For this review, take the finished solid that the model builds, in its own axes (mm). A direction names the side the tool comes from. Coordinates: 2 decimals unless noted, no trailing zeros. Write each loop counter-clockwise with the first axis right and the second up, starting at its lowest first coordinate (ties: lowest second). Pieces come first, ordered by that corner, then holes. Notation, with made-up numbers: M 37,-30.5 L 44,-30.5 A6 cw 44,-21.5 Z; hole C 79.25,55.5 d6. An arc over 180 degrees is marked long. One line per question, with ' | ' between items.
from build123d import *

# Parameters (mm, degrees)
SKETCH1_W           = 200
SKETCH1_H           = 194
BOSS_EXTRUDE1_DEPTH = 8
SKETCH4_R           = 2.4
CUT_EXTRUDE1_DEPTH  = 6
SKETCH5_W           = 200
SKETCH5_H           = 194
SKETCH5_W_2         = 192
SKETCH5_H_2         = 180
BOSS_EXTRUDE4_DEPTH = 60
SKETCH6_W           = 192
SKETCH6_H           = 6
BOSS_EXTRUDE5_DEPTH = 4
SKETCH7_R           = 2.4
CUT_EXTRUDE2_DEPTH  = 6
SKETCH10_R          = 3.9
SKETCH10_R_2        = 7.7
SKETCH10_W          = 12.3
SKETCH10_H          = 19
CUT_EXTRUDE4_DEPTH  = 10
SKETCH16_R          = 5
SKETCH16_R_2        = 5.9
SKETCH16_W          = 13
SKETCH16_H          = 16
CUT_EXTRUDE5_DEPTH  = 10
SKETCH17_W          = 15
SKETCH17_H          = 15
CUT_EXTRUDE6_DEPTH  = 3
SKETCH19_R          = 2.4
CUT_EXTRUDE7_DEPTH  = 5
SKETCH20_R          = 6.5
CUT_EXTRUDE8_DEPTH  = 6
SKETCH22_W          = 35
SKETCH22_H          = 34
CUT_EXTRUDE9_DEPTH  = 4
SKETCH23_W          = 34.5
SKETCH23_H          = 19.9
CUT_EXTRUDE10_DEPTH = 12
CUT_EXTRUDE11_DEPTH = 1
SKETCH25_R          = 2.4
CUT_EXTRUDE12_DEPTH = 5
SKETCH26_W          = 144
SKETCH26_H          = 60
CUT_EXTRUDE13_DEPTH = 287.810041665
SKETCH27_W          = 42.5
SKETCH27_H          = 27.9
SKETCH27_W_2        = 34.5
SKETCH27_H_2        = 19.9
BOSS_EXTRUDE7_DEPTH = 1
FILLET5_R           = 5
BOSS_EXTRUDE8_DEPTH = 3
FILLET6_R           = 5
SKETCH30_R          = 2.4
CUT_EXTRUDE14_DEPTH = 5
SKETCH32_R          = 1.65
CUT_EXTRUDE15_DEPTH = 15
FILLET7_R           = 5
FILLET8_R           = 5
FILLET9_R           = 5
FILLET10_R          = 25
SKETCH33_W          = 206
SKETCH33_H          = 200
BOSS_EXTRUDE9_DEPTH = 5


with BuildPart() as part:
    # Sketch1 → Boss-Extrude1 (new body)
    with BuildSketch(Plane(origin=(0, 0, 0), x_dir=(1, 0, 0), z_dir=(0, 1, 0))):
        with Locations((100, -97)):
            Rectangle(SKETCH1_W, SKETCH1_H)
    extrude(amount=BOSS_EXTRUDE1_DEPTH)

    # Sketch4 → Cut-Extrude1 (cut)
    with BuildSketch(Plane(origin=(0, 8, 0), x_dir=(1, 0, 0), z_dir=(0, 1, 0))):
        with Locations(Location((9.25, -31.25, 0), (0, 0, 270))):
            Circle(SKETCH4_R)
        with Locations(Location((95.25, -31.25, 0), (0, 0, 270))):
            Circle(SKETCH4_R)
        with Locations(Location((95.25, -162.75, 0), (0, 0, 90))):
            Circle(SKETCH4_R)
        with Locations(Location((9.25, -162.75, 0), (0, 0, 90))):
            Circle(SKETCH4_R)
        with Locations(Location((190.75, -162.75, 0), (0, 0, 270))):
            Circle(SKETCH4_R)
        with Locations(Location((104.75, -162.75, 0), (0, 0, 270))):
            Circle(SKETCH4_R)
        with Locations(Location((104.75, -31.25, 0), (0, 0, 90))):
            Circle(SKETCH4_R)
        with Locations(Location((190.75, -31.25, 0), (0, 0, 90))):
            Circle(SKETCH4_R)
    extrude(amount=-CUT_EXTRUDE1_DEPTH, mode=Mode.SUBTRACT)

    # Sketch5 → Boss-Extrude4 (add)
    with BuildSketch(Plane(origin=(0, 8, 0), x_dir=(1, 0, 0), z_dir=(0, 1, 0))):
        with Locations((100, -97)):
            Rectangle(SKETCH5_W, SKETCH5_H)
        with Locations((100, -97)):
            Rectangle(SKETCH5_W_2, SKETCH5_H_2, mode=Mode.SUBTRACT)
    extrude(amount=BOSS_EXTRUDE4_DEPTH)

    # Sketch6 → Boss-Extrude5 (add)
    with BuildSketch(Plane.XY.offset(7)):
        with Locations((100, 65)):
            Rectangle(SKETCH6_W, SKETCH6_H)
    boss_extrude5 = extrude(amount=BOSS_EXTRUDE5_DEPTH)

    # Sketch7 → Cut-Extrude2 (cut)
    with BuildSketch(Plane(origin=(0, 68, 0), x_dir=(1, 0, 0), z_dir=(0, 1, 0))):
        with Locations(Location((12.5, -4, 0), (0, 0, 270))):
            Circle(SKETCH7_R)
        with Locations(Location((62.5, -4, 0), (0, 0, 270))):
            Circle(SKETCH7_R)
        with Locations(Location((187.5, -4, 0), (0, 0, 270))):
            Circle(SKETCH7_R)
        with Locations(Location((137.5, -4, 0), (0, 0, 270))):
            Circle(SKETCH7_R)
    cut_extrude2 = extrude(amount=-CUT_EXTRUDE2_DEPTH, mode=Mode.SUBTRACT)

    # Mirror3: Boss-Extrude5 across plane
    add(boss_extrude5.mirror(Plane.XY.offset(97)))

    # Mirror5: Cut-Extrude2 across plane
    add(cut_extrude2.mirror(Plane.XY.offset(97)), mode=Mode.SUBTRACT)

    # Sketch10 → Cut-Extrude4 (cut)
    with BuildSketch(Plane.XY.offset(194)):
        with Locations((18.85, 20)):
            Circle(SKETCH10_R)
        with Locations((170, 32)):
            Circle(SKETCH10_R_2)
        with Locations((40, 20)):
            Rectangle(SKETCH10_W, SKETCH10_H)
    extrude(amount=-CUT_EXTRUDE4_DEPTH, mode=Mode.SUBTRACT)

    # Sketch16 → Cut-Extrude5 (cut)
    with BuildSketch(Plane(origin=(0, 0, 0), x_dir=(-1, 0, 0), z_dir=(0, 0, -1))):
        with Locations((-53, 48)):
            Circle(SKETCH16_R)
        with Locations((-63.5, 37.5)):
            Circle(SKETCH16_R)
        with Locations((-42.5, 37.5)):
            Circle(SKETCH16_R)
        with Locations((-53, 27)):
            Circle(SKETCH16_R)
        with Locations((-18, 48)):
            Circle(SKETCH16_R_2)
        with Locations((-82.2, 42.6)):
            Rectangle(SKETCH16_W, SKETCH16_H)
    extrude(amount=-CUT_EXTRUDE5_DEPTH, mode=Mode.SUBTRACT)

    # Sketch17 → Cut-Extrude6 (cut)
    with BuildSketch(Plane(origin=(0, 0, 0), x_dir=(-1, 0, 0), z_dir=(0, 0, -1))):
        with Locations((-18, 48)):
            Rectangle(SKETCH17_W, SKETCH17_H)
    extrude(amount=-CUT_EXTRUDE6_DEPTH, mode=Mode.SUBTRACT)

    # Sketch19 → Cut-Extrude7 (cut)
    with BuildSketch(Plane.XY.offset(7)):
        with Locations((32.5, 54.4)):
            Circle(SKETCH19_R)
        with Locations((92.5, 54.4)):
            Circle(SKETCH19_R)
        with Locations((92.5, 17.6)):
            Circle(SKETCH19_R)
        with Locations((32.5, 17.6)):
            Circle(SKETCH19_R)
    extrude(amount=-CUT_EXTRUDE7_DEPTH, mode=Mode.SUBTRACT)

    # Sketch20 → Cut-Extrude8 (cut)
    with BuildSketch(Plane.XY.offset(7)):
        with Locations((53, 48)):
            Circle(SKETCH20_R)
        with Locations((42.5, 37.5)):
            Circle(SKETCH20_R)
        with Locations((53, 27)):
            Circle(SKETCH20_R)
        with Locations((63.5, 37.5)):
            Circle(SKETCH20_R)
    extrude(amount=-CUT_EXTRUDE8_DEPTH, mode=Mode.SUBTRACT)

    # Sketch22 → Cut-Extrude9 (cut)
    with BuildSketch(Plane.XY.offset(7)):
        with Locations((163.5, 35.101020514)):
            Rectangle(SKETCH22_W, SKETCH22_H)
    extrude(amount=-CUT_EXTRUDE9_DEPTH, mode=Mode.SUBTRACT)

    # Sketch23 → Cut-Extrude10 (cut)
    with BuildSketch(Plane.XY.offset(3)):
        with Locations((163.5, 36.051020514)):
            Rectangle(SKETCH23_W, SKETCH23_H)
    extrude(amount=-CUT_EXTRUDE10_DEPTH, mode=Mode.SUBTRACT)

    # Sketch24 → Cut-Extrude11 (cut)
    with BuildSketch(Plane.XY.offset(3)):
        Polygon((146.25, 26.101020514), (146.25, 22.001020514), (153.5, 22.001020514), (153.5, 18.101020514), (173.5, 18.101020514), (173.5, 22.001020514), (180.75, 22.001020514), (180.75, 26.101020514), align=None)
    extrude(amount=-CUT_EXTRUDE11_DEPTH, mode=Mode.SUBTRACT)

    # Sketch25 → Cut-Extrude12 (cut)
    with BuildSketch(Plane.XY.offset(7)):
        with Locations((141, 37.101020514)):
            Circle(SKETCH25_R)
        with Locations((186, 37.101020514)):
            Circle(SKETCH25_R)
    extrude(amount=-CUT_EXTRUDE12_DEPTH, mode=Mode.SUBTRACT)

    # Sketch26 → Cut-Extrude13 (cut, through all)
    with BuildSketch(Plane.ZY):
        with Locations((97, 38)):
            Rectangle(SKETCH26_W, SKETCH26_H)
    extrude(amount=-CUT_EXTRUDE13_DEPTH, mode=Mode.SUBTRACT)

    # Sketch27 → Boss-Extrude7 (add)
    with BuildSketch(Plane(origin=(0, 0, 0), x_dir=(-1, 0, 0), z_dir=(0, 0, -1))):
        with Locations((-163.5, 36.051020514)):
            Rectangle(SKETCH27_W, SKETCH27_H)
        with Locations((-163.5, 36.051020514)):
            Rectangle(SKETCH27_W_2, SKETCH27_H_2, mode=Mode.SUBTRACT)
    extrude(amount=BOSS_EXTRUDE7_DEPTH)

    # Fillet5
    fillet5_edges = [part.edges().sort_by_distance(p)[0] for p in [
        (184.75, 50.001020514, -0.5),
        (184.75, 22.101020514, -0.5),
        (142.25, 22.101020514, -0.5),
        (142.25, 50.001020514, -0.5),
    ]]
    fillet(fillet5_edges, radius=FILLET5_R)

    # Sketch28 → Boss-Extrude8 (add)
    with BuildSketch(Plane.ZY.offset(-196)):
        Polygon((25, 68), (11, 68), (11, 62), (7, 62), (7, 38), (11, 38), (25, 38), align=None)
        Polygon((183, 68), (169, 68), (169, 38), (183, 38), (187, 38), (187, 62), (183, 62), align=None)
    boss_extrude8 = extrude(amount=BOSS_EXTRUDE8_DEPTH)

    # Fillet6
    # the kernel refuses this fillet: 5 mm, written as the material it adds along each edge
    with BuildSketch(Plane(origin=(196, 38, 169), x_dir=(-1, 0, 0), z_dir=(0, 0, 1)), Plane(origin=(196, 38, 7), x_dir=(-1, 0, 0), z_dir=(0, 0, 1))) as fillet6_piece_1:
        with BuildLine():
            CenterArc((5, 4.582575695), FILLET6_R, 180, 66.421821522)
            Line((0, 4.582575695), (0, 0))
            Line((0, 0), (3, 0))
        make_face()
    extrude(amount=18)

    # Sketch30 → Cut-Extrude14 (cut)
    with BuildSketch(Plane.ZY.offset(-193)):
        with Locations((18, 60)):
            Circle(SKETCH30_R)
        with Locations((18, 44)):
            Circle(SKETCH30_R)
        with Locations(Location((176, 44, 0), (0, 0, 180))):
            Circle(SKETCH30_R)
        with Locations(Location((176, 60, 0), (0, 0, 180))):
            Circle(SKETCH30_R)
    cut_extrude14 = extrude(amount=-CUT_EXTRUDE14_DEPTH, mode=Mode.SUBTRACT)

    # Sketch32 → Cut-Extrude15 (cut)
    with BuildSketch(Plane.ZY.offset(-198)):
        with Locations((18, 60)):
            Circle(SKETCH32_R)
        with Locations((18, 44)):
            Circle(SKETCH32_R)
        with Locations((176, 44)):
            Circle(SKETCH32_R)
        with Locations((176, 60)):
            Circle(SKETCH32_R)
    cut_extrude15 = extrude(amount=-CUT_EXTRUDE15_DEPTH, mode=Mode.SUBTRACT)

    # Mirror8: Boss-Extrude8, Cut-Extrude14, Cut-Extrude15 across plane
    add(boss_extrude8.mirror(Plane(origin=(100, 0, 0), x_dir=(0, 0, 1), z_dir=(1, 0, 0))))
    add(cut_extrude14.mirror(Plane(origin=(100, 0, 0), x_dir=(0, 0, 1), z_dir=(1, 0, 0))), mode=Mode.SUBTRACT)
    add(cut_extrude15.mirror(Plane(origin=(100, 0, 0), x_dir=(0, 0, 1), z_dir=(1, 0, 0))), mode=Mode.SUBTRACT)

    # Fillet7
    # the kernel refuses this fillet: 5 mm, written as the material it adds along each edge
    with BuildSketch(Plane(origin=(4, 38, 169), x_dir=(0, -1, 0), z_dir=(0, 0, 1))) as fillet7_piece_1_section:
        with BuildLine():
            CenterArc((4.582575695, 5), FILLET7_R, 203.578178478, 66.421821522)
            Line((0, 3), (0, 0))
            Line((0, 0), (4.582575695, 0))
        make_face()
    fillet7_piece_1 = extrude(amount=29.456439237, mode=Mode.PRIVATE)
    fillet7_piece_1 = split(fillet7_piece_1, bisect_by=Plane(origin=(4.808333267, 36.161514318, 194), z_dir=(0, 0, -1)), keep=Keep.TOP, mode=Mode.PRIVATE)
    add(fillet7_piece_1)
    with BuildSketch(Plane(origin=(4, 38, -4.456439237), x_dir=(0, -1, 0), z_dir=(0, 0, 1))) as fillet7_piece_2_section:
        with BuildLine():
            CenterArc((4.582575695, 5), FILLET7_R, 203.578178478, 66.421821522)
            Line((0, 3), (0, 0))
            Line((0, 0), (4.582575695, 0))
        make_face()
    fillet7_piece_2 = extrude(amount=29.456439237, mode=Mode.PRIVATE)
    fillet7_piece_2 = split(fillet7_piece_2, bisect_by=Plane(origin=(4.808333267, 36.161514318, 0), z_dir=(0, 0, 1)), keep=Keep.TOP, mode=Mode.PRIVATE)
    add(fillet7_piece_2)

    # Fillet8
    # the kernel refuses this fillet: 5 mm, written as the material it adds along each edge
    with BuildSketch(Plane(origin=(7, 62, 7), x_dir=(0, -1, 0), z_dir=(1, 0, 0))) as fillet8_piece_1:
        with BuildLine():
            CenterArc((4.898979486, -5), FILLET8_R, 90, 78.463040967)
            Line((0, -4), (0, 0))
            Line((0, 0), (4.898979486, 0))
        make_face()
    extrude(amount=186)

    # Fillet9
    # the kernel refuses this fillet: 5 mm, written as the material it adds along each edge
    with BuildSketch(Plane(origin=(7, 62, 187), x_dir=(0, -1, 0), z_dir=(1, 0, 0))) as fillet9_piece_1:
        with BuildLine():
            CenterArc((4.898979486, 5), FILLET9_R, 191.536959033, 78.463040967)
            Line((0, 4), (0, 0))
            Line((0, 0), (4.898979486, 0))
        make_face()
    extrude(amount=186)

    # Fillet10
    fillet10_edges = [part.edges().sort_by_distance(p)[0] for p in [
        (198, 8, 25),
        (198, 8, 169),
        (2, 8, 169),
        (2, 8, 25),
    ]]
    fillet(fillet10_edges, radius=FILLET10_R)

    # Sketch33 → Boss-Extrude9 (add)
    with BuildSketch(Plane.XZ):
        with Locations((100, 97)):
            Rectangle(SKETCH33_W, SKETCH33_H)
    extrude(amount=BOSS_EXTRUDE9_DEPTH)


solid = part.part
1) Insertion check: pin 1 Ø10.5 at (x, y) = (66, 36.5) entering from +Z; pin 2 Ø7.5 at (y, z) = (44, 18) entering from -X; pin 3 Ø6 at (x, y) = (32.5, 54.4) entering from -Z. Each pin has a flat end and moves straight along its axis. Give the tip position at first contact, or say it passes through.
Responses:
pin 1: z = 194 | pin 2: x = 0 | pin 3: z = 0
2) To check wall thickness, follow line 1 along X through (y, z) = (3.3, 31.25); line 2 along Z through (x, y) = (137, 66); line 3 along Y through (x, z) = (199, 18). State the ranges of each line that lie inside material, in increasing order. Write a range as [from, to].
Responses:
line 1: [0, 6.85], [11.65, 92.85], [97.65, 102.35], [107.15, 188.35], [193.15, 200] | line 2: [0, 1.65], [6.35, 11], [183, 187.65], [192.35, 194] | line 3: [-5, 42.35], [45.65, 58.35], [61.65, 68]
3) Machinability: for faces 3 (the cylindrical face through (34.717, 53.481, 4.535)), 4 (the cylindrical face through (139.88, 65.04, 3.69)), 5 (the cylindrical face through (198.028, 15.129, 32.518)), 6 (the flat face through (75.7, 42, 3)), which of the approach directions +Z, -Z, +X, -X, +Y, -Y give a long, thin tool a straight path to every point of the face, cutting with its end or side? Answer none if there is none.
Responses:
face 3: none | face 4: +Y | face 5: +X, -X, +Y | face 6: -Z
4) We need section A-A on z = 190. State how many separate pieces and enclosed holes the cut face has, then the cut area to 3 significant figures.
Responses:
separate pieces: 1 | enclosed holes: 3 | area: 14,000 mm^2
5) We need section D-D on z = 116. State the section outline as (x, y) points, then the cut area to 3 significant figures.
Responses:
outline: M -3,-5 L 203,-5 L 203,0 L 200,0 L 200,8 L 0,8 L 0,0 L -3,0 Z | area: 2,630 mm^2
6) The part is to be moulded in two halves that separate along Z. For faces 1 (the flat face through (163, 23, 2)), 2 (the cylindrical face through (20.65, 16.54, 190.55)), say which applies: +Z half, -Z half, draft (parallel to the pull), parting line (faces both ways), or undercut.
Responses:
face 1: undercut | face 2: draft
7) We need section C-C on x = 104.75. State the section outline as (y, z) points, then the cut area to 3 significant figures.
Responses:
outline: M -5,-3 L 0,-3 L 0,0 L 68,0 L 68,11 L 62,11 A5 cw 57.1,7 L 8,7 L 8,28.85 L 2,28.85 L 2,33.65 L 8,33.65 L 8,160.35 L 2,160.35 L 2,165.15 L 8,165.15 L 8,187 L 57.1,187 A5 cw 62,183 L 68,183 L 68,194 L 0,194 L 0,197 L -5,197 Z | area: 3,390 mm^2
